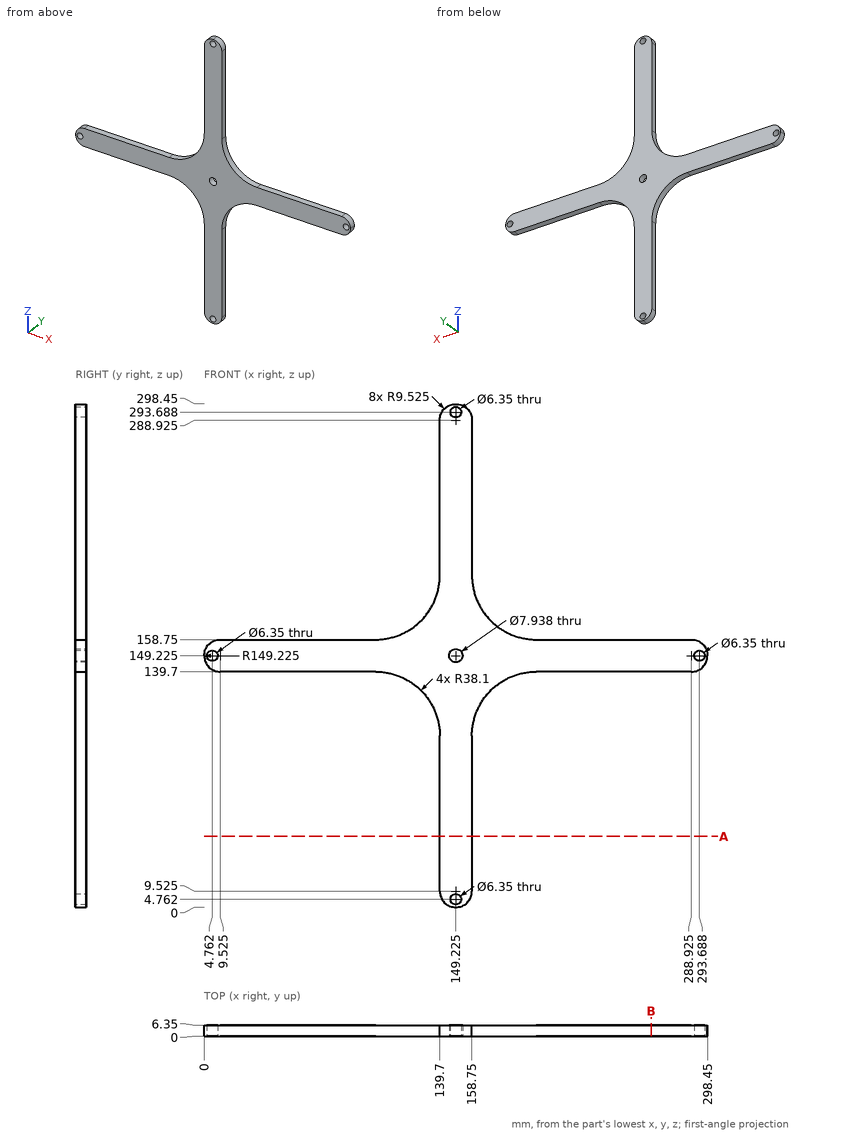
Design review of the part shown in the three views and the two pictorial views. Dimensions are in mm from the part's minimum x, y and z. Coordinates: 2 decimals unless noted, no trailing zeros. Loops run counter-clockwise (first coordinate to the right, second up) from the corner with the lowest first, then second, coordinate; pieces in that order, holes last.
(1) Insertion check: P1, Ø2, axis at x = 71, y = 2.5, coming from the +Z side; P2, Ø8.5, axis at x = 4.76, z = 149.22, coming from the +Y side; P3, Ø1.5, axis at x = 38.5, y = 5.5, coming from the -Z side; P4, Ø1.5, axis at y = 2.5, z = 135, coming from the +X side (1 decimal). Each pin has a flat end and moves straight along its axis. Give the tip position at first contact, or say it passes through.
Determined:
P1: stops at z = 158.75
P2: stops at y = 6.35
P3: stops at z = 139.7
P4: stops at x = 180
(2) Consider section A-A, the plane z = 42. Give the boundary of the cut face in (x, y), plus the area to 3 significant figures.
Determined:
outline: (139.7, 0) - (158.75, 0) - (158.75, 6.35) - (139.7, 6.35) - close
area: 121 mm2
(3) Wall thickness on L1, parallel to Z at x = 50, y = 2.25; L2, parallel to X at y = 4.5, z = 127: over which ranges is each line inside the solid? List them lowest first.
Determined:
L1: z = 139.7 to 158.75
L2: x = 130 to 168.45
(4) Consider section B-B, the plane x = 265. Give the boundary of the cut face in (y, z), plus the area to 3 significant figures.
Determined:
outline: (0, 139.7) - (6.35, 139.7) - (6.35, 158.75) - (0, 158.75) - close
area: 121 mm2
